```python
from build123d import *

# Parameters (mm, degrees)
EXTRUDE_1_DEPTH     = 5
SKETCH_3_R          = 4
CUT_EXTRUDE_1_DEPTH = 49.918299235
CUT_EXTRUDE_2_DEPTH = 49.918299235


with BuildPart() as part:
    # 草图1 → 凸台-拉伸1 (new body)
    with BuildSketch(Plane.XY):
        with BuildLine():
            Line((-4, -6.92820323), (-4, 0))
            Line((-4, 0), (4, 0))
            Line((4, 0), (4, -6.92820323))
            ThreePointArc((4, -6.92820323), (6.92820323, -4), (8, 0))
            ThreePointArc((8, 0), (-4, 6.92820323), (-4, -6.92820323))
        make_face()
        with BuildLine():
            Line((4, 0), (-4, 0))
            Line((-4, 0), (-4, -6.92820323))
            ThreePointArc((-4, -6.92820323), (0, -8), (4, -6.92820323))
            Line((4, -6.92820323), (4, 0))
        make_face()
        with BuildLine():
            ThreePointArc((4, -6.92820323), (0, -8), (-4, -6.92820323))
            Line((-4, -6.92820323), (-4, -33.07179677))
            ThreePointArc((-4, -33.07179677), (0, -32), (4, -33.07179677))
            Line((4, -33.07179677), (4, -6.92820323))
        make_face()
        with BuildLine():
            ThreePointArc((4, -33.07179677), (0, -32), (-4, -33.07179677))
            Line((-4, -33.07179677), (-4, -40))
            Line((-4, -40), (4, -40))
            Line((4, -40), (4, -33.07179677))
        make_face()
        with BuildLine():
            Line((-4, -40), (-4, -33.07179677))
            ThreePointArc((-4, -33.07179677), (-4, -46.92820323), (8, -40))
            ThreePointArc((8, -40), (6.92820323, -36), (4, -33.07179677))
            Line((4, -33.07179677), (4, -40))
            Line((4, -40), (-4, -40))
        make_face()
    extrude(amount=EXTRUDE_1_DEPTH)

    # 草图3 → 切除-拉伸1 (cut, through all)
    with BuildSketch(Plane(origin=(0, 0, 0), x_dir=(-1, 0, 0), z_dir=(0, 0, -1))):
        Circle(SKETCH_3_R)
        with Locations((0, -40)):
            Circle(SKETCH_3_R)
    extrude(amount=-CUT_EXTRUDE_1_DEPTH, mode=Mode.SUBTRACT)

    # 草图4 → 切除-拉伸2 (cut, through all)
    with BuildSketch(Plane(origin=(0, 0, 0), x_dir=(-1, 0, 0), z_dir=(0, 0, -1))):
        with BuildLine():
            Line((1.657955328, -10), (1.657955328, -30))
            ThreePointArc((1.657955328, -30), (0, -31.657955328), (-1.657955328, -30))
            Line((-1.657955328, -30), (-1.657955328, -10))
            ThreePointArc((-1.657955328, -10), (0, -8.342044672), (1.657955328, -10))
        make_face()
    extrude(amount=-CUT_EXTRUDE_2_DEPTH, mode=Mode.SUBTRACT)


solid = part.part
```
For this review, take the finished solid that the model builds, in its own axes (mm). A direction names the side the tool comes from. Round coordinates to 2 decimals unless told otherwise and drop trailing zeros. Write each loop counter-clockwise with the first axis right and the second up, starting at its lowest first coordinate (ties: lowest second). Pieces come first, ordered by that corner, then holes. Notation, with made-up numbers: (-32.5, -9) -> (0.5, -9) arc R14 ccw to (0.5, 0) -> close; hole circle Ø10 at (8.5, 30). An arc over 180 degrees is marked (long way). One line per question, with ' | ' between items. Start each with the question number.
(1) Add section B-B, the plane x = 0. Write out the cut boundary in (y, z), plus the area to 3 significant figures.
(2) Insertion check: P1, Ø2, axis at x = 1, z = 3.5, coming from the -Y side; P2, Ø1.5, axis at y = -21, z = 1.5, coming from the +X side; P3, Ø1, axis at y = -29, z = 2, coming from the -X side; P4, Ø1, axis at x = -1.5, z = 0.5, coming from the +Y side. Each pin has a flat end and moves straight along its axis. Give the tip position at first contact, or say it passes through.
(3) Add section A-A, the plane y = -12.5. Write out the cut boundary in (x, z), plus the area to 3 significant figures.
(4) Tool access review of faces 1 (the face through (-2, -20, 0)), 2 (the face through (4, -20, 2)), 3 (the face through (-1.658, -20, 2)): name each direction out of +Z, -Z, +X, -X, +Y, -Y from which nothing blocks a thin tool from reaching the whole face with its end or side.
(5) Add section D-D, the plane x = -2.5. Write out the cut boundary in (y, z).
(6) Mouldability with a two-part tool opening along Y and no side actions: class faces 4 (the face through (-2, -20, 5)), 5 (the face through (-4, -20, 2)) as released by +Y, released by -Y, zero draft, split by the parting line, or undercut.
(7) Add section C-C, the plane z = 2.45. Write out the cut boundary in (x, y).
(8) For line 1 along Y through (x, z) = (0, 1.5); line 2 along X through (y, z) = (-29, 4.7); line 3 along Y through (x, z) = (-1.25, 4.4), list the stretches that pass through material, from the lowest coordinate up. Write a range as from..to.
Answer list:
1) outline: (-48, 0) -> (-44, 0) -> (-44, 5) -> (-48, 5) -> close; (-36, 0) -> (-31.66, 0) -> (-31.66, 5) -> (-36, 5) -> close; (-8.34, 0) -> (-4, 0) -> (-4, 5) -> (-8.34, 5) -> close; (4, 0) -> (8, 0) -> (8, 5) -> (4, 5) -> close | area: 83.4 mm²
2) P1: y = -48 | P2: x = 4 | P3: x = -4 | P4: y = 7.94
3) outline: (-4, 0) -> (-1.66, 0) -> (-1.66, 5) -> (-4, 5) -> close; (1.66, 0) -> (4, 0) -> (4, 5) -> (1.66, 5) -> close | area: 23.4 mm²
4) face 1: -Z, +X, -X, +Y, -Y | face 2: +Z, -Z, +X | face 3: +Z, -Z
5) outline: (-47.6, 0) -> (-43.12, 0) -> (-43.12, 5) -> (-47.6, 5) -> close; (-36.88, 0) -> (-3.12, 0) -> (-3.12, 5) -> (-36.88, 5) -> close; (3.12, 0) -> (7.6, 0) -> (7.6, 5) -> (3.12, 5) -> close
6) face 4: zero draft | face 5: undercut
7) outline: (-4, -33.07) arc R8 ccw (long way) to (4, -33.07) -> (4, -6.93) arc R8 ccw (long way) to (-4, -6.93) -> close; hole circle Ø8 at (0, -40); hole circle Ø8 at (0, 0); hole (-1.66, -30) arc R1.66 ccw to (1.66, -30) -> (1.66, -10) arc R1.66 ccw to (-1.66, -10) -> close
8) line 1: -48..-44, -36..-31.66, -8.34..-4, 4..8 | line 2: -4..-1.66, 1.66..4 | line 3: -47.9..-43.8, -36.2..-31.09, -8.91..-3.8, 3.8..7.9
